Geometry: see drawing. Coordinates: mm, zero at the bounding-box minimum. A direction names the side the tool comes from. Give positions to 0.01 mm unless a question says otherwise; leave off trailing zeros. Order: outer loops, then holes, each group sorted by start corner. A loop starts at its lowest first (then second) coordinate and runs counter-clockwise, first axis right, second up. Notation, with made-up numbers: (87, 2.25) - (97, 2.25) arc R14 ccw to (97, 15.25) - close; hole circle Ø4 at (-5, 89). An arc over 180 degrees is marked (long way). One line per question, with ' | ' between items. Start each with the question number.
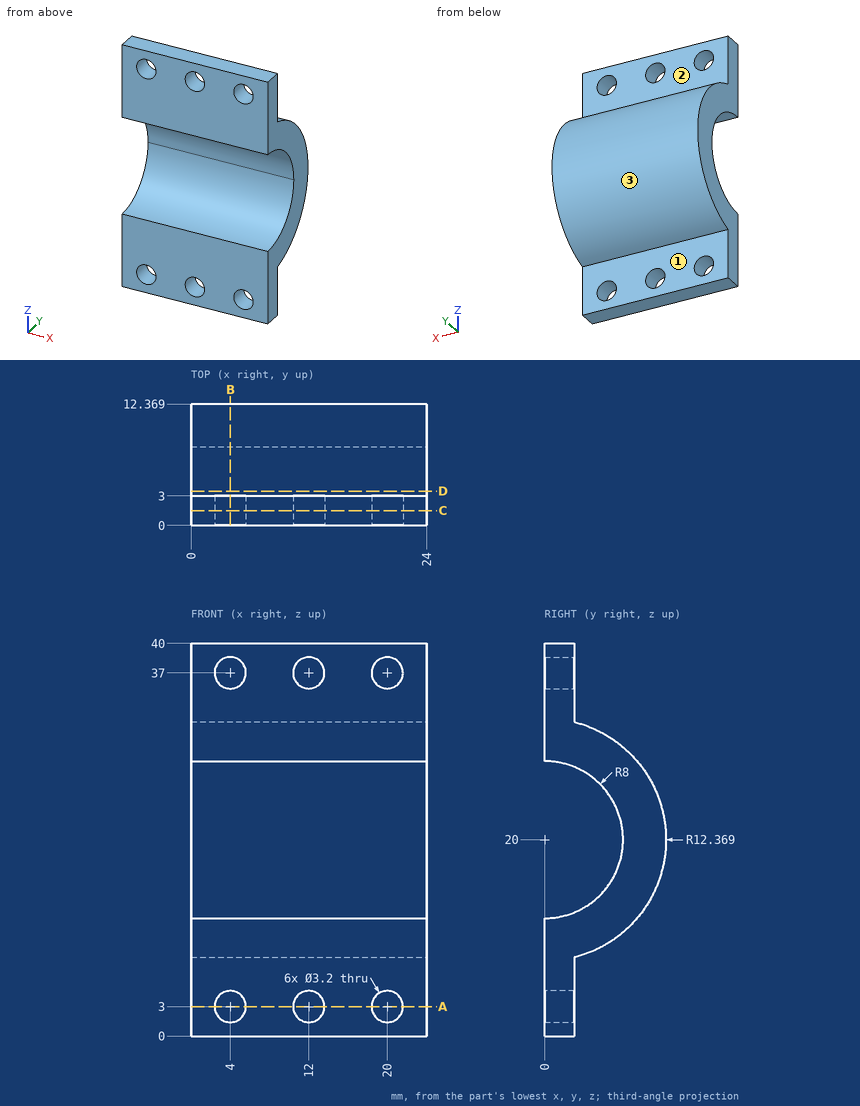
(1) Access query for the marked faces 1, 2 and 3. Directions: +Z, -Z, +X, -X, +Y, -Y. A direction counts if a zero-diameter tool reaches every point of the face in a straight line with its end or side. Return the directions, or none.
(2) Contact query for flat-ended pins moving along their axis: P1, Ø3, axis at x = 5.5, z = 23.5, coming from the -Y side (1 decimal); P2, Ø4, axis at x = 12, z = 3, coming from the -Y side; P3, Ø1, axis at x = 7.5, z = 21.5, coming from the +Y side; P4, Ø6.5, axis at x = 14.5, z = 3.5, coming from the +Y side. Output: stop coordinate, or through.
(3) Cut plane A-A, the plane z = 3. Return the cut outline in (x, y), plus the area to 3 significant figures.
(4) Cut plane C-C, the plane y = 1.5. Return the cut outline in (x, z).
(5) Cut plane B-B, the plane x = 4. Return the cut outline in (y, z).
(6) Cut plane D-D, the plane y = 3.5. Return the cut outline in (x, z), plus the area to 3 significant figures.
(7) Material intervals for line 1 along X through (y, z) = (2.4, 37); line 2 along Z through (x, y) = (11.25, 0.5) (1 decimal); line 3 along Z through (x, y) = (17, 6) (1 decimal), sorted ascending. Write a range as from..to.
Results are:
1) face 1: -Z, +X, -X, +Y | face 2: +Z, +X, -X, +Y | face 3: +X, -X, +Y
2) P1: y = 6.2 | P2: y = 0 | P3: y = 12.33 | P4: y = 3
3) outline: (0, 0) - (2.4, 0) - (2.4, 3) - (0, 3) - close; (5.6, 0) - (10.4, 0) - (10.4, 3) - (5.6, 3) - close; (13.6, 0) - (18.4, 0) - (18.4, 3) - (13.6, 3) - close; (21.6, 0) - (24, 0) - (24, 3) - (21.6, 3) - close | area: 43.2 mm2
4) outline: (0, 0) - (24, 0) - (24, 12.14) - (0, 12.14) - close; (0, 27.86) - (24, 27.86) - (24, 40) - (0, 40) - close; hole circle Ø3.2 at (4, 3); hole circle Ø3.2 at (4, 37); hole circle Ø3.2 at (12, 3); hole circle Ø3.2 at (12, 37); hole circle Ø3.2 at (20, 3); hole circle Ø3.2 at (20, 37)
5) outline: (0, 0) - (3, 0) - (3, 1.4) - (0, 1.4) - close; (0, 4.6) - (3, 4.6) - (3, 8) arc R12.37 ccw to (3, 32) - (3, 35.4) - (0, 35.4) - (0, 28) arc R8 cw to (0, 12) - close; (0, 38.6) - (3, 38.6) - (3, 40) - (0, 40) - close
6) outline: (0, 8.14) - (24, 8.14) - (24, 12.81) - (0, 12.81) - close; (0, 27.19) - (24, 27.19) - (24, 31.86) - (0, 31.86) - close | area: 224 mm2
7) line 1: 0..2.4, 5.6..10.4, 13.6..18.4, 21.6..24 | line 2: 0..1.6, 4.4..12, 28..35.6, 38.4..40 | line 3: 9.2..14.7, 25.3..30.8
